```python
from build123d import *

# Parameters (mm, degrees)
F0_W       = 35
F0_H       = 35
F2_W       = 28
F2_H       = 28
F4_T       = -1.2
F5_R       = 3
F6_DEPTH   = 7
F7_SIZE2   = 3
F7_SIZE    = 6
F7_2_SIZE2 = 3
F7_2_SIZE  = 6
F7_3_SIZE2 = 3
F7_3_SIZE  = 6
F7_4_SIZE2 = 3
F7_4_SIZE  = 6
F10_DEPTH  = 7


# Not quite as in the source:
# - a feature names something its author has since deleted; it is built from what else it names


with BuildPart() as f3:
    # F0 (on Top) → F3 section 0
    with BuildSketch(Plane.XY):
        Rectangle(F0_W, F0_H)
    # F2 (on offset) → F3 section 1
    with BuildSketch(Plane.XY.offset(7)):
        Rectangle(F2_W, F2_H)
    loft()

    # F4
    f4_openings = [f3.faces().sort_by_distance(p)[0] for p in [
        (0, 0, 7),
        (0, 0, 0),
    ]]
    offset(amount=F4_T, openings=f4_openings)


with BuildPart() as f6:
    # F5 (on Top) → F6 (new body, through all)
    with BuildSketch(Plane.XY):
        with BuildLine():
            Line((-16.2, -0.8), (-4.1231056256, -0.8))
            ThreePointArc((-4.1231056256, -0.8), (-2.9768706674, -2.9628096513), (-0.8195121951, -4.1192717514))
            Line((-0.8195121951, -4.1192717514), (-0.8195121951, -16.2))
            Line((-0.8195121951, -16.2), (0.8195121951, -16.2))
            Line((0.8195121951, -16.2), (0.8195121951, -4.1192717514))
            ThreePointArc((0.8195121951, -4.1192717514), (2.9768706674, -2.9628096513), (4.1231056256, -0.8))
            Line((4.1231056256, -0.8), (16.2, -0.8))
            Line((16.2, -0.8), (16.2, 0.8195121951))
            Line((16.2, 0.8195121951), (4.1192717514, 0.8195121951))
            ThreePointArc((4.1192717514, 0.8195121951), (2.9628096513, 2.9768706674), (0.8, 4.1231056256))
            Line((0.8, 4.1231056256), (0.8, 16.2))
            Line((0.8, 16.2), (-0.8, 16.2))
            Line((-0.8, 16.2), (-0.8, 4.1231056256))
            ThreePointArc((-0.8, 4.1231056256), (-2.969848481, 2.969848481), (-4.1231056256, 0.8))
            Line((-4.1231056256, 0.8), (-16.2, 0.8))
            Line((-16.2, 0.8), (-16.2, -0.8))
        make_face()
        Circle(F5_R, mode=Mode.SUBTRACT)
    extrude(amount=F6_DEPTH)

    # F7
    f7_edges = [f6.edges().sort_by_distance(p)[0] for p in [
        (-16.2, 0, 7),
    ]]
    f7_side = f6.faces().sort_by_distance((-16.2, 0, 3.5))[0]
    chamfer(f7_edges, length=F7_SIZE, length2=F7_SIZE2, reference=f7_side)

    # F7#2
    f7_2_edges = [f6.edges().sort_by_distance(p)[0] for p in [
        (0, 16.2, 7),
    ]]
    f7_2_side = f6.faces().sort_by_distance((0, 16.2, 3.5))[0]
    chamfer(f7_2_edges, length=F7_2_SIZE, length2=F7_2_SIZE2, reference=f7_2_side)

    # F7#3
    f7_3_edges = [f6.edges().sort_by_distance(p)[0] for p in [
        (16.2, 0.009756, 7),
    ]]
    f7_3_side = f6.faces().sort_by_distance((16.2, 0.009756, 3.5))[0]
    chamfer(f7_3_edges, length=F7_3_SIZE, length2=F7_3_SIZE2, reference=f7_3_side)

    # F7#4
    f7_4_edges = [f6.edges().sort_by_distance(p)[0] for p in [
        (0, -16.2, 7),
    ]]
    f7_4_side = f6.faces().sort_by_distance((0, -16.2, 3.5))[0]
    chamfer(f7_4_edges, length=F7_4_SIZE, length2=F7_4_SIZE2, reference=f7_4_side)


with BuildPart() as f3_1:
    add(f3.part)

    # F8: union F6
    add(f6.part)

    # F9 (on face) → F10 (join, through all)
    with BuildSketch(Plane.XY.offset(7)):
        with BuildLine():
            Line((0.6612347815, 0.8790725588), (-0.3595485903, 2.9783762038))
            ThreePointArc((-0.3595485903, 2.9783762038), (-0.8973940811, 2.8626358244), (-1.4050598491, 2.6506238549))
            Line((-1.4050598491, 2.6506238549), (0.6612347815, 0.8790725588))
        make_face()
        with BuildLine():
            Line((-0.430681777, 1.0121823981), (-2.7591237497, 1.1778098887))
            ThreePointArc((-2.7591237497, 1.1778098887), (-2.9278123863, 0.6541518408), (-2.9980375188, 0.1084944043))
            Line((-2.9980375188, 0.1084944043), (-0.430681777, 1.0121823981))
        make_face()
        with BuildLine():
            Line((-1.0919165585, 0.1331098393), (-2.3995751593, -1.800566315))
            ThreePointArc((-2.3995751593, -1.800566315), (-2.0304183052, -2.2084839836), (-1.5929776697, -2.5421294507))
            Line((-1.5929776697, -2.5421294507), (-1.0919165585, 0.1331098393))
        make_face()
        with BuildLine():
            Line((-0.6612347815, -0.8790725588), (0.3595485903, -2.9783762038))
            ThreePointArc((0.3595485903, -2.9783762038), (0.8973940811, -2.8626358244), (1.4050598491, -2.6506238549))
            Line((1.4050598491, -2.6506238549), (-0.6612347815, -0.8790725588))
        make_face()
        with BuildLine():
            ThreePointArc((2.7591237497, -1.1778098887), (2.9278123863, -0.6541518408), (2.9980375188, -0.1084944043))
            Line((2.9980375188, -0.1084944043), (0.430681777, -1.0121823981))
            Line((0.430681777, -1.0121823981), (2.7591237497, -1.1778098887))
        make_face()
        with BuildLine():
            ThreePointArc((2.3995751593, 1.800566315), (2.0304183052, 2.2084839836), (1.5929776697, 2.5421294507))
            Line((1.5929776697, 2.5421294507), (1.0919165585, -0.1331098393))
            Line((1.0919165585, -0.1331098393), (2.3995751593, 1.800566315))
        make_face()
    extrude(amount=-F10_DEPTH)


solid = f3_1.part
```
Input: part model. Units: mm. Frame: model coordinates. A direction names the side the tool comes from. Coordinates: 2 decimals unless noted, no trailing zeros. Use a Markdown table: item, result. Add a question column.
1) Draft query along Y for faces 1 (the cylindrical face through (2.87, 0.88, 3.45)), 2 (the flat face through (-0.1, 2.1, 7)). Return one class per face: +Y half, -Y half, draft (parallel to the pull), parting line (faces both ways), or undercut.
2) Pin query (flat end, axial travel): P1, Ø2, axis at y = 7, z = 4, coming from the +X side; P2, Ø2, axis at x = 10.5, z = 3.5, coming from the -Y side; P3, Ø2, axis at y = 12, z = 1.5, coming from the +X side. Return the tip coordinate at first contact, or that it passes through.
3) Line query: L1, parallel to X at y = 5, z = 4; L2, parallel to Y at x = -1, z = 6; L3, parallel to Y at x = -5, z = 4.25 (3 decimals). Output: solid intervals per line, ascending. Write a range as from..to.
4) Set-up query: faces 3 (the flat face through (2, -3, 0)), 4 (the cylindrical face through (-2.95, 2.99, 3.45)), 5 (the flat face through (14.384, -6.88, 3.549)). Return all of +Z, -Z, +X, -X, +Y, -Y with unobstructed straight access to the full face (end or side cutting, diameter ignored); none if empty.
5) Section A-A, the plane y = -12. Give the number of separate pieces and of enclosed holes in the cut face, plus the area to 3 significant figures.
Answer below:
| question | item | result |
|---|---|---|
| 1 | face 1 | undercut |
| 1 | face 2 | draft |
| 2 | P1 | x = 16 |
| 2 | P2 | y = -16.25 |
| 2 | P3 | x = 17.25 |
| 3 | L1 | -15.5..-14.16, -0.8..0.8, 14.16..15.5 |
| 3 | L2 | -14.5..-13.16, -4.08..-2.83, 0.81..1.05, 2.3..4.08, 13.16..14.5 |
| 3 | L3 | -15.375..-14.033, -0.8..0.8, 14.033..15.375 |
| 4 | face 3 | -Z, +X, -X, +Y, -Y |
| 4 | face 4 | +Z, -Z |
| 4 | face 5 | -Z |
| 5 | separate pieces | 3 |
| 5 | enclosed holes | 0 |
| 5 | area | 30.3 mm2 |
